```python
from build123d import *

# Parameters (mm, degrees)
SKETCH1_W           = 138
SKETCH1_H           = 43.5
BOSS_EXTRUDE1_DEPTH = 41.5
CUT_EXTRUDE1_DEPTH  = 0.5
CUT_EXTRUDE2_DEPTH  = 0.5
FILLET1_R           = 4
FILLET2_R           = 1
SKETCH5_R           = 1.635
BOSS_EXTRUDE2_DEPTH = 10


with BuildPart() as part:
    # Sketch1 → Boss-Extrude1 (new body)
    with BuildSketch(Plane(origin=(0, 0, -15), x_dir=(-1, 0, 0), z_dir=(0, 0, -1))):
        with Locations((0, -0.25)):
            Rectangle(SKETCH1_W, SKETCH1_H)
    extrude(amount=-BOSS_EXTRUDE1_DEPTH)

    # Sketch2 → Cut-Extrude1 (cut)
    with BuildSketch(Plane(origin=(69, 0, 0), x_dir=(0, 0, -1), z_dir=(1, 0, 0))):
        with BuildLine():
            Line((-21.3125, 8.0625), (-21.3125, -8.5625))
            ThreePointArc((-21.3125, -8.5625), (-18.969354249, -14.219354249), (-13.3125, -16.5625))
            Line((-13.3125, -16.5625), (1.8125, -16.5625))
            ThreePointArc((1.8125, -16.5625), (7.469354249, -14.219354249), (9.8125, -8.5625))
            Line((9.8125, -8.5625), (9.8125, 8.0625))
            ThreePointArc((9.8125, 8.0625), (7.469354249, 13.719354249), (1.8125, 16.0625))
            Line((1.8125, 16.0625), (-13.3125, 16.0625))
            ThreePointArc((-13.3125, 16.0625), (-18.969354249, 13.719354249), (-21.3125, 8.0625))
        make_face()
    extrude(amount=-CUT_EXTRUDE1_DEPTH, mode=Mode.SUBTRACT)

    # Sketch3 → Cut-Extrude2 (cut)
    with BuildSketch(Plane.ZY.offset(69)):
        with BuildLine():
            Line((13.3125, 16.0625), (-1.8125, 16.0625))
            ThreePointArc((-1.8125, 16.0625), (-7.469354249, 13.719354249), (-9.8125, 8.0625))
            Line((-9.8125, 8.0625), (-9.8125, -8.5625))
            ThreePointArc((-9.8125, -8.5625), (-7.469354249, -14.219354249), (-1.8125, -16.5625))
            Line((-1.8125, -16.5625), (13.3125, -16.5625))
            ThreePointArc((13.3125, -16.5625), (18.969354249, -14.219354249), (21.3125, -8.5625))
            Line((21.3125, -8.5625), (21.3125, 8.0625))
            ThreePointArc((21.3125, 8.0625), (18.969354249, 13.719354249), (13.3125, 16.0625))
        make_face()
    extrude(amount=-CUT_EXTRUDE2_DEPTH, mode=Mode.SUBTRACT)

    # Fillet1
    fillet1_edges = [part.edges().sort_by_distance(p)[0] for p in [
        (-69, -0.25, 26.5),
        (69, -0.25, 26.5),
        (-69, -0.25, -15),
        (69, -0.25, -15),
    ]]
    fillet(fillet1_edges, radius=FILLET1_R)

    # Fillet2
    fillet2_edges = [part.edges().sort_by_distance(p)[0] for p in [
        (0, -22, -15),
        (0, 21.5, -15),
        (-69, 21.5, 5.75),
        (0, 21.5, 26.5),
        (69, 21.5, 5.75),
        (67.828427125, 21.5, 25.328427125),
        (67.828427125, 21.5, -13.828427125),
        (-67.828427125, 21.5, 25.328427125),
        (-67.828427125, 21.5, -13.828427125),
        (-69, -22, 5.75),
        (69, -22, 5.75),
        (0, -22, 26.5),
        (67.828427125, -22, 25.328427125),
        (67.828427125, -22, -13.828427125),
        (-67.828427125, -22, 25.328427125),
        (-67.828427125, -22, -13.828427125),
    ]]
    fillet(fillet2_edges, radius=FILLET2_R)

    # Sketch5 → Boss-Extrude2 (add)
    with BuildSketch(Plane.ZY.offset(-69)):
        with Locations((-7.474307757, -18.480417137)):
            Circle(SKETCH5_R)
        with Locations((-3.551789479, -18.480417137)):
            Circle(SKETCH5_R)
        with Locations((1.821805343, -18.480417137)):
            Circle(SKETCH5_R)
        with Locations((5.75, -18.480417137)):
            Circle(SKETCH5_R)
    extrude(amount=-BOSS_EXTRUDE2_DEPTH)


solid = part.part
```
Verification items for the finished model (mm, model axes). A direction names the side the tool comes from. Coordinates: 2 decimals unless noted, no trailing zeros. Order: outer loops, then holes, each group sorted by start corner. A loop starts at its lowest first (then second) coordinate and runs counter-clockwise, first axis right, second up. Notation, with made-up numbers: (19.5, -10) -> (68.5, -10) arc R16 ccw to (68.5, 3) -> close; hole circle Ø5 at (28.5, 8). An arc over 180 degrees is marked (long way). Put each result on its own line as item: value. Start each with the question number.
1) Go/stop test with flat-tipped pins: pin 1 (0.6 mm diameter, centred on x = 68.5, y = 2.5, fed in from +Z); pin 2 (0.6 mm diameter, centred on x = -69, z = 9, fed in from +Y); pin 3 (3 mm diameter, centred on y = -5.5, z = 13, fed in from +X). Record where each tip stops, or that it passes through.
2) Material ranges on L1, parallel to X at y = -9, z = -10; L2, parallel to Z at x = 65.5, y = 7; L3, parallel to X at y = -13, z = 12.5, recorded low to high.
3) Cross-section at B-B (y = 1.5). Enter the section's corners in (x, z).
4) Cross-section at C-C (y = 17.5). Enter the section's corners in (x, z), plus the area to 3 significant figures.
5) Release check for a two-part mould opening along Z. For faces 4 (the flat face through (1, 21.5, 5)), 5 (the cylindrical face through (-68.75, -14.16, -7.53)), 6 (the flat face through (1, 0, -15)) record: pulls with the +Z half, pulls with the -Z half, needs draft (parallel to the pull), parting line crosses it, or undercut.
6) Cross-section at A-A (z = 10). Enter the section's corners in (x, y).
7) Tool access check on faces 1 (the cylindrical face through (73.93, -17.989, -5.915)), 2 (the flat face through (1, -22, 5)), 3 (the flat face through (-68.5, 0, 6)). Record the directions out of +Z, -Z, +X, -X, +Y, -Y that give a thin tool (end or side, any length) a straight path to the whole face; none if there is none.
Geometry check:
1. pin 1: stops at z = 24.9
1. pin 2: stops at y = 21.21
1. pin 3: stops at x = 68.5
2. L1: x = -69 to 69
2. L2: z = -14.97 to 26.47
2. L3: x = -68.5 to 68.5
3. outline: (-69, -11) arc R4 ccw to (-65, -15) -> (65, -15) arc R4 ccw to (69, -11) -> (69, -9.81) -> (68.5, -9.81) -> (68.5, 21.31) -> (69, 21.31) -> (69, 22.5) arc R4 ccw to (65, 26.5) -> (-65, 26.5) arc R4 ccw to (-69, 22.5) -> (-69, 21.31) -> (-68.5, 21.31) -> (-68.5, -9.81) -> (-69, -9.81) -> close
4. outline: (-69, -11) arc R4 ccw to (-65, -15) -> (65, -15) arc R4 ccw to (69, -11) -> (69, 22.5) arc R4 ccw to (65, 26.5) -> (-65, 26.5) arc R4 ccw to (-69, 22.5) -> close
4. area: 5,710 mm^2
5. face 4: needs draft
5. face 5: undercut
5. face 6: pulls with the -Z half
6. outline: (-69, -21) arc R1 ccw to (-68, -22) -> (68, -22) arc R1 ccw to (69, -21) -> (69, -16.56) -> (68.5, -16.56) -> (68.5, 16.06) -> (69, 16.06) -> (69, 20.5) arc R1 ccw to (68, 21.5) -> (-68, 21.5) arc R1 ccw to (-69, 20.5) -> (-69, 16.06) -> (-68.5, 16.06) -> (-68.5, -16.56) -> (-69, -16.56) -> close
7. face 1: +X
7. face 2: +Z, -Z, +X, -X, -Y
7. face 3: -X
